Source: three-view drawing plus pictorial views. Frame: mm from the lowest corner of the part. Coordinates: 2 decimals unless noted, no trailing zeros. Write each loop counter-clockwise with the first axis right and the second up, starting at its lowest first coordinate (ties: lowest second). Pieces come first, ordered by that corner, then holes. Notation, with made-up numbers: (81, -26.75) -> (98, -26.75) arc R14 cw to (98, -16.75) -> close; hole circle Ø6 at (47.25, -39.5). An arc over 180 degrees is marked (long way). Write item = value, one per line.
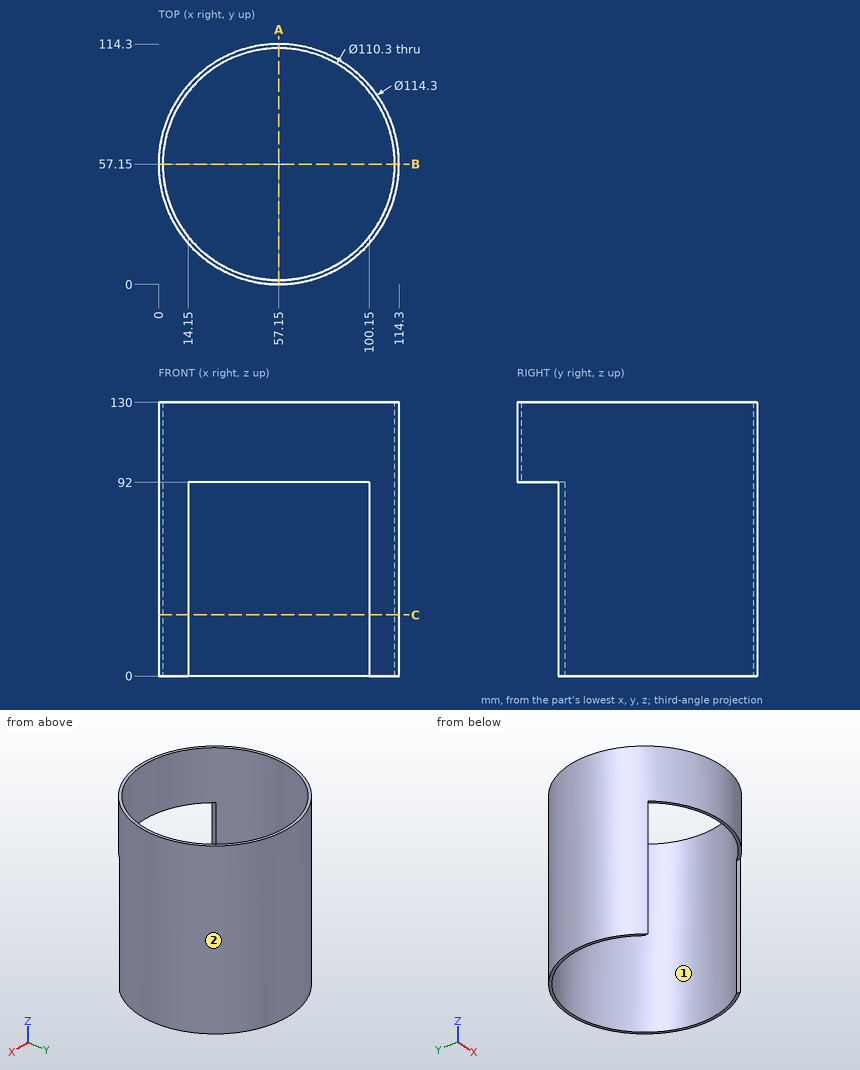
1) Cut plane B-B, the plane y = 57.15. Output: boundary loops of the cut face in (x, z).
Answer block:
outline = (0, 0) -> (2, 0) -> (2, 130) -> (0, 130) -> close; (112.3, 0) -> (114.3, 0) -> (114.3, 130) -> (112.3, 130) -> close
2) Cut plane C-C, the plane z = 29. Output: boundary loops of the cut face in (x, y), and give its area (3 significant figures).
Answer block:
outline = (14.15, 19.51) -> (14.15, 22.62) arc R55.15 cw (long way) to (100.15, 22.62) -> (100.15, 19.51) arc R57.15 ccw (long way) to start
area = 510 mm2
3) Material intervals for probe 1 along X at (y, z) = (57.15, 86.5); probe 2 along Y at (x, z) = (100.5, 117.5), sorted ascending. Write a range as [from, to].
Answer block:
probe_1 = [0, 2], [112.3, 114.3]
probe_2 = [19.91, 23.06], [91.24, 94.39]
4) Cut plane A-A, the plane x = 57.15. Output: boundary loops of the cut face in (y, z), and give its area (3 significant figures).
Answer block:
outline = (0, 92) -> (2, 92) -> (2, 130) -> (0, 130) -> close; (112.3, 0) -> (114.3, 0) -> (114.3, 130) -> (112.3, 130) -> close
area = 336 mm2
5) Pull-direction query (X, two-part tool) for the marked faces 1 and 2; classes: +X half, -X half, draft (parallel to the pull), parting line (faces both ways), or undercut.
Answer block:
face_1 = undercut
face_2 = parting line
6) First-contact query: pin 1 Ø1 at (y, z) = (24, 29) entering from -X; pin 2 Ø10 at (y, z) = (15, 25.5) entering from -X; pin 3 Ø10 at (y, z) = (67.5, 31) entering from -X. Flat tips, straight axial feed; report the tip coordinate or a pass-through.
Answer block:
pin_1 = 10.24
pin_2 = 13.72
pin_3 = 0.25
